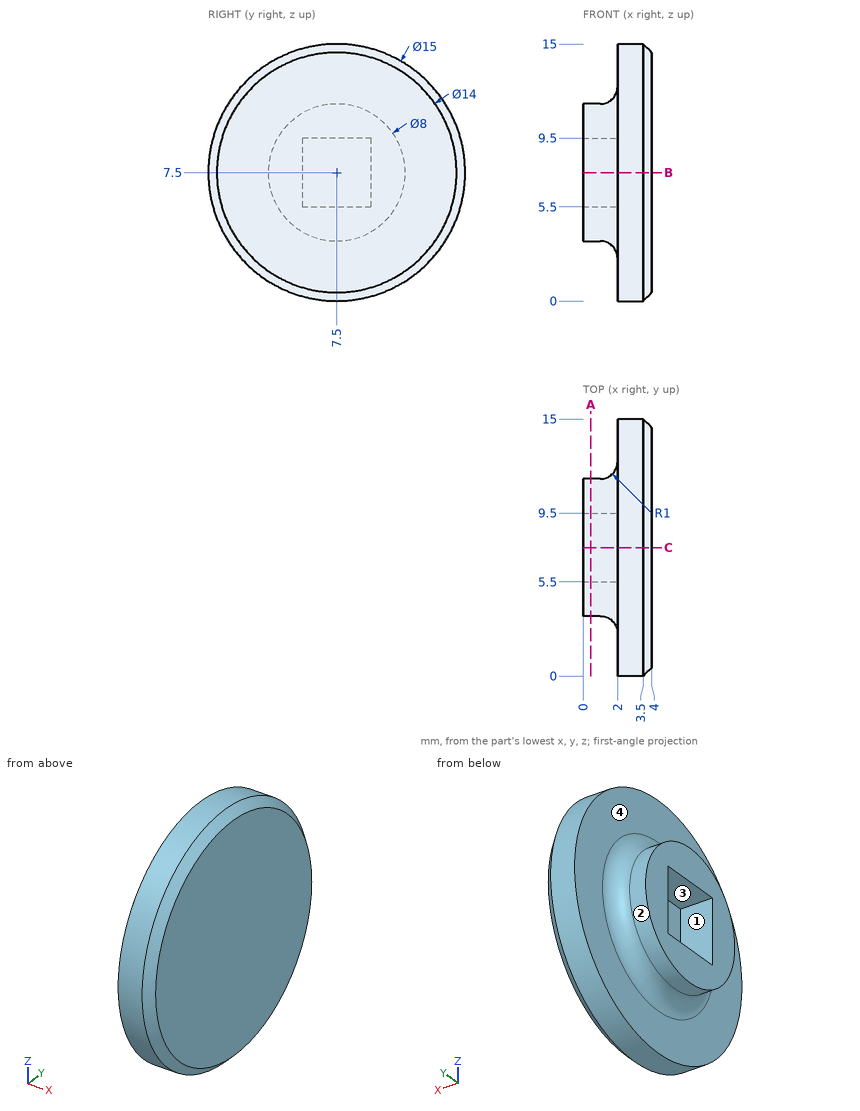
Could you check a few things on this drawing? It's one solid part, dimensions in mm from its lowest x, y, z. Round coordinates to 2 decimals unless told otherwise and drop trailing zeros. Loops run counter-clockwise (first coordinate to the right, second up) from the corner with the lowest first, then second, coordinate; pieces in that order, holes last.
Q1. Thinking about a two-plate mould opening in Z: for the marked faces 1, 2, 3 and 4, which applies, pulls with the +Z half, pulls with the -Z half, needs draft (parallel to the pull), parting line crosses it, or undercut?
Q2. I want a section at A-A (x = 0.45). Write out the boundary of the cut face in (y, z), and give its area (3 significant figures).
Q3. I want a section at B-B (z = 7.5). Write out the boundary of the cut face in (x, y).
Q4. For P1, Ø4.5, axis at y = 7, z = 7.5, coming from the -X side; P2, Ø1, axis at x = 2.5, y = 9, coming from the -Z side; P3, Ø1.6, axis at x = 1, z = 8, coming from the -Y side; P4, Ø0.6, axis at x = 1, z = 7, coming from the +Y side, each with a flat end and sliding along its axis, tell me the tip position at first contact or that it passes through.
Q5. Please list where these lines run through material, in increasing order: L1, parallel to Y at x = 1.4, z = 9; L2, parallel to X at y = 1.5, z = 8.25; L3, parallel to Z at x = 0.85, y = 7.75.
Answer below:
1. face 1: undercut
1. face 2: parting line crosses it
1. face 3: undercut
1. face 4: needs draft
2. outline: circle Ø8 at (7.5, 7.5); hole (5.5, 5.5) - (9.5, 5.5) - (9.5, 9.5) - (5.5, 9.5) - close
2. area: 34.3 mm2
3. outline: (0, 3.5) - (1, 3.5) arc R1 cw to (2, 2.5) - (2, 0) - (3.5, 0) - (4, 0.5) - (4, 14.5) - (3.5, 15) - (2, 15) - (2, 12.5) arc R1 cw to (1, 11.5) - (0, 11.5) - (0, 9.5) - (2, 9.5) - (2, 5.5) - (0, 5.5) - close
4. P1: stops at x = 0
4. P2: stops at z = 0.07
4. P3: stops at y = 3.13
4. P4: stops at y = 11.52
5. L1: y = 3.7 to 5.5, 9.5 to 11.3
5. L2: x = 2 to 4
5. L3: z = 3.51 to 5.5, 9.5 to 11.49
